Autodesk Inventor part; units mm, degrees
ref_plane "YZ Plane" through (0, 0, 0) normal (1, 0, 0) x (0, 1, 0)
ref_plane "XZ Plane" through (0, 0, 0) normal (0, 1, 0) x (-1, 0, 0)
ref_plane "XY Plane" through (0, 0, 0) normal (0, 0, 1) x (1, 0, 0)
sketch "Náčrt1" plane through (0, 0, 0) normal (0, 1, 0) x (-1, 0, 0)
  line L0 (0, 0) -> (-75, 0)
  line L1 (-75, 0) -> (-75, -60)
  line L2 (-75, -60) -> (0, -60)
  line L3 (0, -60) -> (0, 0)
  line L4 (2, 2) -> (-77, 2)
  line L5 (-77, 2) -> (-77, -62)
  line L6 (-77, -62) -> (2, -62)
  line L7 (2, -62) -> (2, 2)
  dimension "d0" = 2
  dimension "d1" = 2
  dimension "d2" = 2
  dimension "d3" = 2
  dimension "d4" = 75
  dimension "d5" = 60
extrude "Vysunutí1" add sketch "Náčrt1" along normal blind 2 contours L3 L2 L1 L0 | L7 L6 L5 L4
sketch "Náčrt2" plane through (0, 2, 0) normal (0, 1, 0) x (1, 0, 0)
  circle A0 centre (1.5, 1.5) radius 1.5
  circle A1 centre (1.5, 58.5) radius 1.5
  circle A2 centre (73.5, 58.5) radius 1.5
  circle A3 centre (73.5, 1.5) radius 1.5
  line L0 (-2, 62) -> (-2, -2)
  line L1 (-2, -2) -> (77, -2)
  line L2 (77, 62) -> (-2, 62)
  line L3 (77, -2) -> (77, 62)
  point P0 (0, 0)
  dimension "d8" = 3
  dimension "d9" = 3
  dimension "d10" = 3
  dimension "d11" = 3
  dimension "d12" = 3.5
  dimension "d13" = 3.5
  dimension "d14" = 3.5
  dimension "d15" = 3.5
  dimension "d16" = 3.5
  dimension "d17" = 3.5
  dimension "d18" = 3.5
  dimension "d19" = 3.5
extrude "Vysunutí2" cut sketch "Náčrt2" against normal blind 2 contours A0 | A1 | A2 | A3
chamfer "Zkosení1" distance 0.5 angle 45 4 edges at (0, 2, -1.5) (0, 2, -58.5) (72, 2, -58.5) (72, 2, -1.5)
fillet "Zaoblení1" radius 2 4 edges at (77, 1, 2) (77, 1, -62) (-2, 1, -62) (-2, 1, 2)
sketch "Náčrt3" plane through (0, 2, 0) normal (0, 1, 0) x (1, 0, 0)
  line L0 (28.2, 22.75) -> (47.2, 22.75)
  line L1 (47.2, 22.75) -> (47.2, 37.25)
  line L2 (47.2, 37.25) -> (28.2, 37.25)
  line L3 (28.2, 37.25) -> (28.2, 22.75)
  circle A0 centre (30.75, 25.3) radius 1.35
  circle A1 centre (30.75, 34.7) radius 1.35
  line L4 (0, -2) -> (75, -2)
  line L5 (-2, 60) -> (-2, 0)
  line L6 (77, 0) -> (77, 60)
  line L7 (27.2, 21.75) -> (48.2, 21.75)
  line L8 (48.2, 21.75) -> (48.2, 38.25)
  line L9 (48.2, 38.25) -> (27.2, 38.25)
  line L10 (27.2, 38.25) -> (27.2, 21.75)
  point P0 (0, 0)
  dimension "d26" = 14.5
  dimension "d27" = 19
  dimension "d28" = 2.55
  dimension "d29" = 2.7
  dimension "d30" = 2.55
  dimension "d31" = 2.7
  dimension "d32" = 2.55
  dimension "d33" = 2.55
  dimension "d34" = 24.75
  dimension "d35" = 30.2
  dimension "d36" = 79
  dimension "d37" = 1
  dimension "d38" = 1
  dimension "d39" = 1
  dimension "d40" = 1
  dimension "d47" = 9.4
extrude "Vysunutí3" add sketch "Náčrt3" along normal blind 1.2 contours L10 L9 L8 L7
extrude "Vysunutí4" add sketch "Náčrt3" along normal blind 1.2 contours A0 | A1
sketch "Náčrt4" plane through (48.2, 2, -21.75) normal (1, 0, 0) x (0, 0, -1)
  line L0 (1, 0) -> (1, 1.2)
  line L1 (15.5, 0) -> (15.5, 1.2)
  line L2 (1, 1.2) -> (15.5, 1.2)
  line L3 (15.5, 1.2) -> (15.5, 0)
  line L4 (15.5, 0) -> (1, 0)
  line L5 (1, 0) -> (1, 1.2)
  point P0 (-21.75, -2)
extrude "Vysunutí5" cut sketch "Náčrt4" against normal blind 1.2
equation "\"d1\" = d0"
equation "\"d2\" = d0"
equation "\"d3\" = d0"
equation "\"d9\" = d8"
equation "\"d10\" = d8"
equation "\"d11\" = d8"
equation "\"d14\" = d12"
equation "\"d15\" = d12"
equation "\"d16\" = d12"
equation "\"d17\" = d12"
equation "\"d18\" = d12"
equation "\"d19\" = d12"
equation "\"d32\" = d30"
equation "\"d33\" = d28"
equation "\"d38\" = d37"
equation "\"d39\" = d37"
equation "\"d40\" = d37"
properties part number "BH1750-viko"
Check sheet for the modelled part. Datum: model origin and axes. Units: mm. A direction names the side the tool comes from. Round coordinates to 2 decimals unless told otherwise and drop trailing zeros. Loops run counter-clockwise (first coordinate to the right, second up) from the corner with the lowest first, then second, coordinate; pieces in that order, holes last. Notation, with made-up numbers: (34, -16) -> (68, -16) arc R9 ccw to (68, -10) -> close; hole circle Ø8 at (76, 55). An arc over 180 degrees is marked (long way). Put each result on its own line as item: value. Start each with the question number.
1. Access from +Z, -Z, +X, -X, +Y, -Y to the whole of each face (thin tool, end or side, straight path). Record for faces 5 (the face through (74.93, 0.76, -58.95)), 6 (the face through (31.476, 2.592, -33.562)).
2. Section check A-A (z = -58.5). Enter the section's corners in (x, y).
3. Scan lines: probe 1 along X at (y, z) = (1.15, -1.5); probe 2 along Z at (x, y) = (1.5, 1.1); probe 3 along Y at (x, z) = (40, -0.5). Record each from-to range of solid material in increasing order.
4. Section check D-D (x = 30.75). Enter the section's corners in (y, z), plus the area to 3 significant figures.
5. Gauge pin test, flat end, axial feed: pin 1 (0.5 mm diameter, centred on y = 2.5, z = -22.5, fed in from +X). Record the tip position at first contact, or that the pin passes through.
6. Section check B-B (x = 73.5). Enter the section's corners in (y, z), plus the area to 4 significant figures.
7. Section check C-C (y = 2.65). Enter the section's corners in (x, z).
8. Draft check along Z on faces 1 (the face through (31, 3.2, -25)), 2 (the face through (31.997, 2.592, -25.817)), 3 (the face through (76.43, 1.01, -61.4)), 4 (the face through (-1.43, 1.01, 1.4)). Enter one of: +Z half, -Z half, draft (parallel to the pull), parting line (faces both ways), or undercut.
Findings:
1. face 5: +Y, -Y
1. face 6: +Y
2. outline: (-2, 0) -> (0, 0) -> (0, 1.5) -> (-0.5, 2) -> (-2, 2) -> close; (3, 0) -> (72, 0) -> (72, 1.5) -> (71.5, 2) -> (3.5, 2) -> (3, 1.5) -> close; (75, 0) -> (77, 0) -> (77, 2) -> (75.5, 2) -> (75, 1.5) -> close
3. probe 1: x = -2 to 0, 3 to 72, 75 to 77
3. probe 2: z = -62 to -60, -57 to -3, 0 to 2
3. probe 3: y = 0 to 2
4. outline: (0, -62) -> (2, -62) -> (2, -38.25) -> (3.2, -38.25) -> (3.2, -37.25) -> (2, -37.25) -> (2, -36.05) -> (3.2, -36.05) -> (3.2, -33.35) -> (2, -33.35) -> (2, -26.65) -> (3.2, -26.65) -> (3.2, -23.95) -> (2, -23.95) -> (2, -22.75) -> (3.2, -22.75) -> (3.2, -21.75) -> (2, -21.75) -> (2, 2) -> (0, 2) -> close
4. area: 137 mm^2
5. pin 1: stops at x = 48.2
6. outline: (0, -62) -> (2, -62) -> (2, -60.5) -> (1.5, -60) -> (0, -60) -> close; (0, -57) -> (1.5, -57) -> (2, -56.5) -> (2, -3.5) -> (1.5, -3) -> (0, -3) -> close; (0, 0) -> (1.5, 0) -> (2, 0.5) -> (2, 2) -> (0, 2) -> close
6. area: 115.5 mm^2
7. outline: (27.2, -38.25) -> (48.2, -38.25) -> (48.2, -37.25) -> (28.2, -37.25) -> (28.2, -22.75) -> (48.2, -22.75) -> (48.2, -21.75) -> (27.2, -21.75) -> close; circle Ø2.7 at (30.75, -34.7); circle Ø2.7 at (30.75, -25.3)
8. face 1: draft
8. face 2: undercut
8. face 3: -Z half
8. face 4: +Z half
